Here's how the part is built. I have some questions about the finished solid (model axes, mm). Give positions to 0.01 mm unless a question says otherwise; leave off trailing zeros. Order: outer loops, then holes, each group sorted by start corner. A loop starts at its lowest first (then second) coordinate and runs counter-clockwise, first axis right, second up. Notation, with made-up numbers: M 8.25,10.5 L 37.25,10.5 A28 ccw 37.25,44.5 Z; hole C 34.25,10 d6. An arc over 180 degrees is marked long. Use one line per item in the form item = value.
from build123d import *

# Parameters (mm, degrees)
SKETCH_1_R      = 1.5
SKETCH_1_R_2    = 2.5
SKETCH_1_W      = 10
SKETCH_1_H      = 20
EXTRUDE_1_DEPTH = 4


with BuildPart() as part:
    # 草圖1 → 填料-伸長1 (new body)
    with BuildSketch(Plane(origin=(0, 4, 0), x_dir=(1, 0, 0), z_dir=(0, 1, 0))):
        Polygon((-75, 160.5), (-90, 190.5), (-110, 190.5), (-110, -190.5), (110, -190.5), (110, 190.5), (90, 190.5), (75, 160.5), align=None)
        with Locations((79.5, -32.62)):
            Circle(SKETCH_1_R, mode=Mode.SUBTRACT)
        with Locations((79.5, -140.62)):
            Circle(SKETCH_1_R, mode=Mode.SUBTRACT)
        with Locations((-83, -6)):
            Circle(SKETCH_1_R_2, mode=Mode.SUBTRACT)
        with Locations((42, -21)):
            Circle(SKETCH_1_R_2, mode=Mode.SUBTRACT)
        with Locations((42, -146)):
            Circle(SKETCH_1_R_2, mode=Mode.SUBTRACT)
        with Locations((-83, -146)):
            Circle(SKETCH_1_R_2, mode=Mode.SUBTRACT)
        with Locations((-83, 119)):
            Circle(SKETCH_1_R_2, mode=Mode.SUBTRACT)
        with Locations((42, -6)):
            Circle(SKETCH_1_R_2, mode=Mode.SUBTRACT)
        with Locations((-83, -21)):
            Circle(SKETCH_1_R_2, mode=Mode.SUBTRACT)
        with Locations((42, 119)):
            Circle(SKETCH_1_R_2, mode=Mode.SUBTRACT)
        with BuildLine():
            Line((-104, 1.5), (-102, 1.5))
            ThreePointArc((-102, 1.5), (-100.5, 0), (-102, -1.5))
            Line((-102, -1.5), (-104, -1.5))
            ThreePointArc((-104, -1.5), (-105.5, 0), (-104, 1.5))
        make_face(mode=Mode.SUBTRACT)
        with BuildLine():
            Line((102, -116), (104, -116))
            ThreePointArc((104, -116), (105.5, -117.5), (104, -119))
            Line((104, -119), (102, -119))
            ThreePointArc((102, -119), (100.5, -117.5), (102, -116))
        make_face(mode=Mode.SUBTRACT)
        with BuildLine():
            Line((102, 1.5), (104, 1.5))
            ThreePointArc((104, 1.5), (105.5, 0), (104, -1.5))
            Line((104, -1.5), (102, -1.5))
            ThreePointArc((102, -1.5), (100.5, 0), (102, 1.5))
        make_face(mode=Mode.SUBTRACT)
        with BuildLine():
            Line((102, 119), (104, 119))
            ThreePointArc((104, 119), (105.5, 117.5), (104, 116))
            Line((104, 116), (102, 116))
            ThreePointArc((102, 116), (100.5, 117.5), (102, 119))
        make_face(mode=Mode.SUBTRACT)
        with BuildLine():
            Line((-104, -116), (-102, -116))
            ThreePointArc((-102, -116), (-100.5, -117.5), (-102, -119))
            Line((-102, -119), (-104, -119))
            ThreePointArc((-104, -119), (-105.5, -117.5), (-104, -116))
        make_face(mode=Mode.SUBTRACT)
        with BuildLine():
            Line((-104, 119), (-102, 119))
            ThreePointArc((-102, 119), (-100.5, 117.5), (-102, 116))
            Line((-102, 116), (-104, 116))
            ThreePointArc((-104, 116), (-105.5, 117.5), (-104, 119))
        make_face(mode=Mode.SUBTRACT)
        Polygon((-85.5, 3.5), (-85.5, 109.5), (-73.5, 121.5), (32.5, 121.5), (44.5, 109.5), (44.5, 3.5), (32.5, -8.5), (-73.5, -8.5), align=None, mode=Mode.SUBTRACT)
        Polygon((-85.5, -30.5), (-73.5, -18.5), (32.5, -18.5), (44.5, -30.5), (44.5, -136.5), (32.5, -148.5), (-73.5, -148.5), (-85.5, -136.5), align=None, mode=Mode.SUBTRACT)
        with Locations((-95, 99.5)):
            Rectangle(SKETCH_1_W, SKETCH_1_H, mode=Mode.SUBTRACT)
        with Locations((54, 99.5)):
            Rectangle(SKETCH_1_W, SKETCH_1_H, mode=Mode.SUBTRACT)
        with Locations((54, -40.5)):
            Rectangle(SKETCH_1_W, SKETCH_1_H, mode=Mode.SUBTRACT)
        with Locations((-95, -40.5)):
            Rectangle(SKETCH_1_W, SKETCH_1_H, mode=Mode.SUBTRACT)
    extrude(amount=-EXTRUDE_1_DEPTH)


solid = part.part
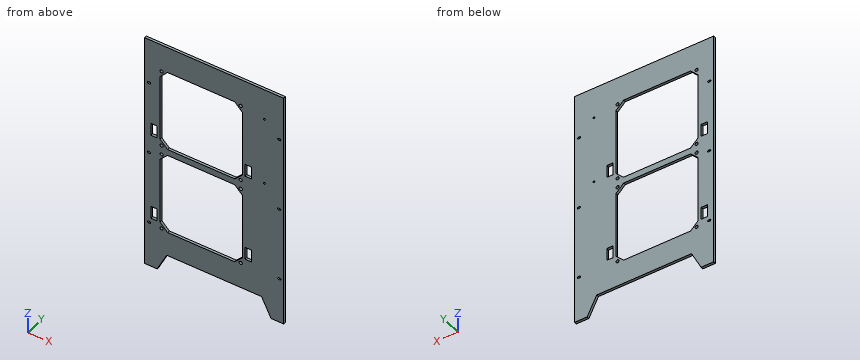
Q1. I want a section at C-C on y = 1.05. State how many separate pieces and enclosed holes the cut face has, then the cut area to 3 significant figures.
Found:
separate_pieces = 1
enclosed_holes = 22
area = 44,600 mm²
Q2. I need wall thicknesses on L1, parallel to X at y = 1.7, z = 32.62; L2, parallel to Z at x = -38, y = 0.55; L3, parallel to X at y = 1.3, z = -103. Which ranges of each line are inside material? Lowest first, please.
Found:
L1 = -110 to -100, -90 to -85.5, 44.5 to 49, 59 to 78, 81 to 110
L2 = -160.5 to -121.5, 8.5 to 18.5, 148.5 to 190.5
L3 = -110 to -100, -90 to -85.5, 44.5 to 49, 59 to 110
Q3. I want a section at D-D on x = 64.5. Write out the boundary of the cut face in (y, z), then the cut area to 3 significant figures.
Found:
outline = M 0,-160.5 L 4,-160.5 L 4,190.5 L 0,190.5 Z
area = 1,400 mm²
Q4. I want a section at B-B on z = -69.5. Write out the boundary of the cut face in (x, y), then the cut area to 3 significant figures.
Found:
outline = M -110,0 L -85.5,0 L -85.5,4 L -110,4 Z; M 44.5,0 L 110,0 L 110,4 L 44.5,4 Z
area = 360 mm²
Q5. I want a section at A-A on x = -59. Write out the boundary of the cut face in (y, z).
Found:
outline = M 0,-160.5 L 4,-160.5 L 4,-121.5 L 0,-121.5 Z; M 0,8.5 L 4,8.5 L 4,18.5 L 0,18.5 Z; M 0,148.5 L 4,148.5 L 4,190.5 L 0,190.5 Z
Q6. I'm going to push flat-ended pins straight in: pin 1 Ø6 at (x, z) = (-83, 146) entering from +Y; pin 2 Ø2 at (x, y) = (52.5, 1.5) entering from -Z. Where does each tip first touch, or does it pass through?
Found:
pin_1 = 4
pin_2 = -160.5
